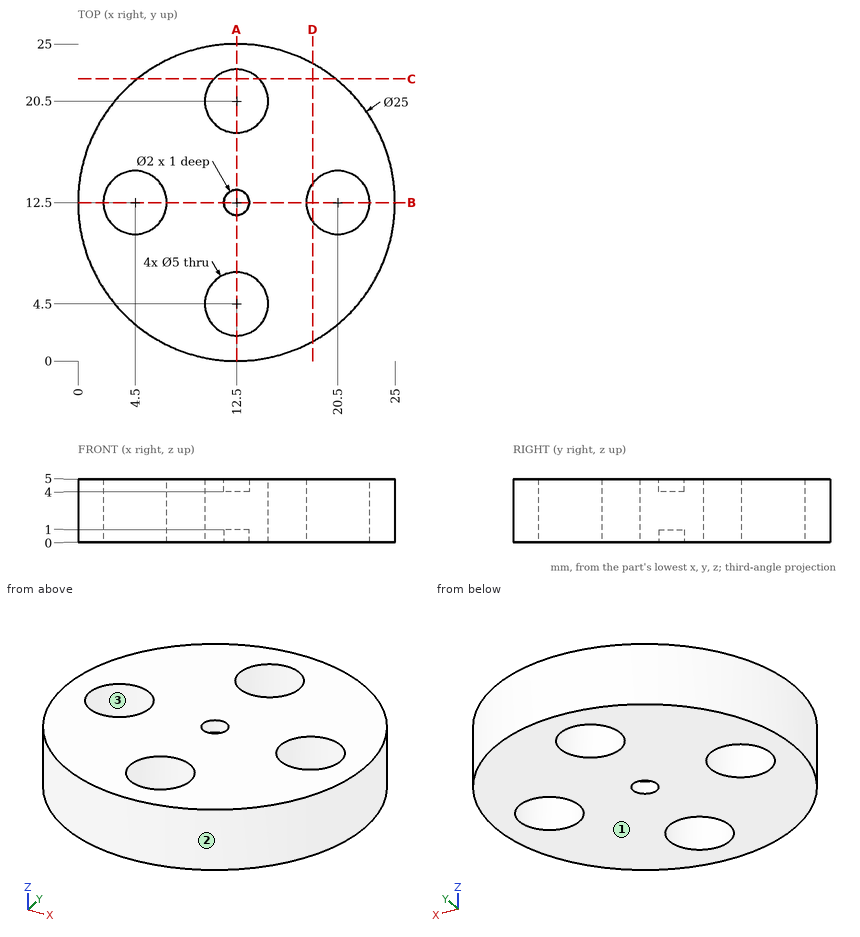
The drawing under review shows one solid part. Ordinate dimensions are in mm from its lowest x, y, z. Coordinates: 2 decimals unless noted, no trailing zeros. Order: outer loops, then holes, each group sorted by start corner. A loop starts at its lowest first (then second) coordinate and runs counter-clockwise, first axis right, second up. Notation, with made-up numbers: (42, 53.5) -> (49, 53.5) arc R15 ccw to (49, 58.5) -> close; hole circle Ø8 at (37, 26). An arc over 180 degrees is marked (long way). Answer in a Markdown table with one row per item. Add a question column.
Item 1: Clearance check with flat-ended pins moving along their axes: pin 1 (4.5 mm diameter, centred on x = 12.5, y = 20.5, fed in from -Z); pin 2 (1 mm diameter, centred on x = 12.5, y = 12.5, fed in from +Z); pin 3 (3 mm diameter, centred on x = 7, z = 1.5, fed in from -Y); pin 4 (3 mm diameter, centred on y = 17.5, z = 4, fed in from +X). State where each tip first meets the part, or that it passes through.
Item 2: We need section D-D on x = 18.5. Write out the cut boundary in (y, z), plus the area to 3 significant figures.
Item 3: We need section C-C on y = 22.25. Write out the cut boundary in (x, z), plus the area to 3 significant figures.
Item 4: We need section A-A on x = 12.5. Write out the cut boundary in (y, z).
Item 5: Mouldability with a two-part tool opening along Y and no side actions: class the marked faces 1, 2 and 3 as +Y half, -Y half, draft (parallel to the pull), parting line (faces both ways), or undercut.
Item 6: To check wall thickness, follow probe 1 along Y at (x, z) = (12.5, 1.85); probe 2 along Y at (x, z) = (12.5, 4.4); probe 3 along X at (y, z) = (10.75, 1.95). State the ranges of each line that lie inside material, in increasing order.
Final values:
| question | item | result |
|---|---|---|
| 1 | pin 1 | passes through |
| 1 | pin 2 | stops at z = 4 |
| 1 | pin 3 | stops at y = 0.66 |
| 1 | pin 4 | stops at x = 24.5 |
| 2 | outline | (1.53, 0) -> (11, 0) -> (11, 5) -> (1.53, 5) -> close; (14, 0) -> (23.47, 0) -> (23.47, 5) -> (14, 5) -> close |
| 2 | area | 94.7 mm2 |
| 3 | outline | (4.68, 0) -> (10.71, 0) -> (10.71, 5) -> (4.68, 5) -> close; (14.29, 0) -> (20.32, 0) -> (20.32, 5) -> (14.29, 5) -> close |
| 3 | area | 60.4 mm2 |
| 4 | outline | (0, 0) -> (2, 0) -> (2, 5) -> (0, 5) -> close; (7, 0) -> (11.5, 0) -> (11.5, 1) -> (13.5, 1) -> (13.5, 0) -> (18, 0) -> (18, 5) -> (13.5, 5) -> (13.5, 4) -> (11.5, 4) -> (11.5, 5) -> (7, 5) -> close; (23, 0) -> (25, 0) -> (25, 5) -> (23, 5) -> close |
| 5 | face 1 | draft |
| 5 | face 2 | parting line |
| 5 | face 3 | undercut |
| 6 | probe 1 | y = 0 to 2, 7 to 18, 23 to 25 |
| 6 | probe 2 | y = 0 to 2, 7 to 11.5, 13.5 to 18, 23 to 25 |
| 6 | probe 3 | x = 0.12 to 2.71, 6.29 to 18.71, 22.29 to 24.88 |
